The model under review builds one solid part; all positions refer to its coordinate system, in mm. A direction names the side the tool comes from. Round coordinates to 2 decimals unless told otherwise and drop trailing zeros. Order: outer loops, then holes, each group sorted by start corner. A loop starts at its lowest first (then second) coordinate and runs counter-clockwise, first axis right, second up. Notation, with made-up numbers: (-33.5, 5) - (-0.5, 5) arc R32 ccw to (-0.5, 31) - close; hole circle Ø11 at (-4, 22). An arc over 180 degrees is marked (long way). One line per question, with ' | ' between items. Start each with the question number.
Item 1: Insertion check: pin 1 Ø0.9 at (y, z) = (38.5, 5.5) entering from -X; pin 2 Ø1.5 at (x, z) = (-15, 5.5) entering from -Y; pin 3 Ø0.9 at (y, z) = (8, 5) entering from +X. Each pin has a flat end and moves straight along its axis. Give the tip position at first contact, or say it passes through.
Item 2: Draft analysis for pull direction Y (two halves, no side actions). For faces 1 (the face through (-13, 42.6, 3)), 2 (the face through (-23.8, 13, 5)), 3 (the face through (-13, 44.6, 5)), state which applies: +Y half, -Y half, draft (parallel to the pull), parting line (faces both ways), or undercut.
Item 3: For L1, parallel to Y at x = -7, z = 4.5; L2, parallel to X at y = 14.5, z = 5; L3, parallel to X at y = 20.5, z = 2.75, list the stretches that pass through material, from the lowest coordinate up. Write a range as [from, to].
Item 4: Add section C-C on x = -8. State the section outline as (y, z) points.
Item 5: Tool access review of faces 4 (the face through (-13, 27, 5)), 5 (the face through (-13, 4, 3)), 6 (the face through (-13, 2, 5)), 7 (the face through (-1.8, 13, 5)): name each direction out of +Z, -Z, +X, -X, +Y, -Y from which nothing blocks a thin tool from reaching the whole face with its end or side.
Item 6: Add section B-B on y = 35. State the section outline as (x, z) points, and give its area (3 significant figures).
Item 7: Add section A-A on z = 5.75. State the section outline as (x, y) points.
Item 8: Add section D-D on z = 3. State the section outline as (x, y) points, and give its area (3 significant figures).
from build123d import *

# Parameters (mm, degrees)
F0_W     = 31.6
F0_H     = 57.9
F0_W_2   = 25.6
F0_H_2   = 51.9
F0_W_3   = 22
F0_H_3   = 22
F0_W_4   = 17.6
F0_H_4   = 17.6
F0_W_5   = 18
F0_H_5   = 18
F0_W_6   = 13.6
F0_H_6   = 13.6
F2_DEPTH = 4
F3_START = 4
F3_DEPTH = 3
F4_SIZE  = 2


with BuildPart() as f2:
    # F0 (on Top) → F2 (new body)
    with BuildSketch(Plane.XY):
        with Locations((-12.8, 25.95)):
            Rectangle(F0_W, F0_H)
        with Locations((-12.8, 25.95)):
            Rectangle(F0_W_2, F0_H_2, mode=Mode.SUBTRACT)
        with Locations((-12.8, 25.95)):
            Rectangle(F0_W_2, F0_H_2)
        with Locations((-12.8, 13)):
            Rectangle(F0_W_3, F0_H_3, mode=Mode.SUBTRACT)
        with Locations((-12.8, 35.8)):
            Rectangle(F0_W_4, F0_H_4, mode=Mode.SUBTRACT)
        with Locations((-12.8, 13)):
            Rectangle(F0_W_3, F0_H_3)
        with Locations((-12.8, 13)):
            Rectangle(F0_W_5, F0_H_5, mode=Mode.SUBTRACT)
        with Locations((-12.8, 35.8)):
            Rectangle(F0_W_4, F0_H_4)
        with Locations((-12.8, 35.8)):
            Rectangle(F0_W_6, F0_H_6, mode=Mode.SUBTRACT)
    extrude(amount=F2_DEPTH)

    # F0 (on Top) → F3 (join)
    with BuildSketch(Plane.XY.offset(F3_START)):
        with Locations((-12.8, 35.8)):
            Rectangle(F0_W_4, F0_H_4)
        with Locations((-12.8, 35.8)):
            Rectangle(F0_W_6, F0_H_6, mode=Mode.SUBTRACT)
        with Locations((-12.8, 13)):
            Rectangle(F0_W_3, F0_H_3)
        with Locations((-12.8, 13)):
            Rectangle(F0_W_5, F0_H_5, mode=Mode.SUBTRACT)
    extrude(amount=F3_DEPTH)

    # F4
    f4_edges = [f2.edges().sort_by_distance(p)[0] for p in [
        (-28.6, 25.95, 0),
        (-12.8, -3, 0),
        (3, 25.95, 0),
        (-12.8, 54.9, 0),
    ]]
    chamfer(f4_edges, length=F4_SIZE)


solid = f2.part
Determined:
1) pin 1: x = -21.6 | pin 2: y = 2 | pin 3: x = -1.8
2) face 1: undercut | face 2: draft | face 3: +Y half
3) L1: [2, 4], [22, 24], [27, 29], [42.6, 44.6] | L2: [-23.8, -21.8], [-3.8, -1.8] | L3: [-28.6, -21.8], [-3.8, 3]
4) outline: (-3, 2) - (-1, 0) - (4, 0) - (4, 7) - (2, 7) - (2, 4) - (-3, 4) - close; (22, 0) - (29, 0) - (29, 7) - (27, 7) - (27, 4) - (24, 4) - (24, 7) - (22, 7) - close; (42.6, 0) - (52.9, 0) - (54.9, 2) - (54.9, 4) - (44.6, 4) - (44.6, 7) - (42.6, 7) - close
5) face 4: +Z, +X, -X | face 5: +Z, -Z | face 6: +Z, +X, -X, -Y | face 7: +Z, +X, +Y, -Y
6) outline: (-28.6, 2) - (-26.6, 0) - (-19.6, 0) - (-19.6, 7) - (-21.6, 7) - (-21.6, 4) - (-28.6, 4) - close; (-6, 0) - (1, 0) - (3, 2) - (3, 4) - (-4, 4) - (-4, 7) - (-6, 7) - close | area: 80.0 mm2
7) outline: (-23.8, 2) - (-1.8, 2) - (-1.8, 24) - (-23.8, 24) - close; (-21.6, 27) - (-4, 27) - (-4, 44.6) - (-21.6, 44.6) - close; hole (-21.8, 4) - (-3.8, 4) - (-3.8, 22) - (-21.8, 22) - close; hole (-19.6, 29) - (-6, 29) - (-6, 42.6) - (-19.6, 42.6) - close
8) outline: (-28.6, -3) - (3, -3) - (3, 54.9) - (-28.6, 54.9) - close; hole (-21.8, 4) - (-3.8, 4) - (-3.8, 22) - (-21.8, 22) - close; hole (-19.6, 29) - (-6, 29) - (-6, 42.6) - (-19.6, 42.6) - close | area: 1,320 mm2
